from build123d import *

# Parameters (mm, degrees)
F1_DEPTH = 16


with BuildPart() as f1:
    # F0 (on Front) → F1 (new body)
    with BuildSketch(Plane.XZ):
        with BuildLine():
            ThreePointArc((0, 55), (16.109127, 16.109127), (55, 0))
            Line((55, 0), (195, 0))
            ThreePointArc((195, 0), (233.890873, 16.109127), (250, 55))
            Line((250, 55), (250, 545))
            ThreePointArc((250, 545), (233.890873, 583.890873), (195, 600))
            Line((195, 600), (125, 600))
            Line((125, 600), (90, 525))
            Line((90, 525), (0, 525))
            Line((0, 525), (0, 55))
        make_face()
        with BuildLine():
            ThreePointArc((48, 172), (50.928932, 179.071068), (58, 182))
            Line((58, 182), (190, 182))
            ThreePointArc((190, 182), (197.071068, 179.071068), (200, 172))
            Line((200, 172), (200, 40))
            ThreePointArc((200, 40), (197.071068, 32.928932), (190, 30))
            Line((190, 30), (58, 30))
            ThreePointArc((58, 30), (50.928932, 32.928932), (48, 40))
            Line((48, 40), (48, 172))
        make_face(mode=Mode.SUBTRACT)
    extrude(amount=F1_DEPTH)


solid = f1.part
Here's how the part is built. I have some questions about the finished solid (model axes, mm). A direction names the side the tool comes from. Give positions to 0.01 mm unless a question says otherwise; leave off trailing zeros. Order: outer loops, then holes, each group sorted by start corner. A loop starts at its lowest first (then second) coordinate and runs counter-clockwise, first axis right, second up. Notation, with made-up numbers: (-8, 77.25) -> (-2, 77.25) arc R15 ccw to (-2, 81.25) -> close; hole circle Ø11 at (-21.75, 2.5). An arc over 180 degrees is marked (long way). Use a Markdown table: item, result. Add a question column.
Item 1: Imagine slicing it at D-D on z = 533.5. Please give me the cut outline in (x, y).
Item 2: I need wall thicknesses on line 1 (Z direction, x = 63.5, y = -12.5); line 2 (Z direction, x = 174, y = -14.25); line 3 (X direction, y = -9.75, z = 35.5). Which ranges of each line are inside material? Lowest first, please.
Item 3: For faces 4 (the face through (123, 0, 304)), 5 (the face through (46, -8, 525)), 6 (the face through (125, -8, 30)), which set-ups out of +Z, -Z, +X, -X, +Y, -Y let a thin tool reach every point of the face, with its end or its side?
Item 4: If we mould it in two halves opening along X, with no side actions, what happens to faces 1 (the face through (160, -8, 600)), 2 (the face through (233.461, -7.888, 15.684)), 3 (the face through (197.15, -7.89, 33.01))? For each: pulls with the +X half, pulls with the -X half, needs draft (parallel to the pull), parting line crosses it, or undercut.
Item 5: Imagine slicing it at A-A on x = 77.5. Please give me the cut outline in (y, z), plus the area to 3 significant figures.
Item 6: Imagine slicing it at B-B on z = 99. Please give me the cut outline in (x, y).
Item 7: Imagine slicing it at C-C on y = -3.25. Please give me the cut outline in (x, z).
Item 8: Will these pins go through, and if not, where does the flat tip stop? pin 1 (1 mm diameter, centred on x = 119.5, y = -9, fed in from +Z); pin 2 (5 mm diameter, centred on x = 26, y = -7.5, fed in from +Z).
Data:
| question | item | result |
|---|---|---|
| 1 | outline | (93.97, -16) -> (250, -16) -> (250, 0) -> (93.97, 0) -> close |
| 2 | line 1 | z = 0 to 30, 182 to 525 |
| 2 | line 2 | z = 0 to 30, 182 to 600 |
| 2 | line 3 | x = 3.57 to 49.07, 198.93 to 246.43 |
| 3 | face 4 | +Z, -Z, +X, -X, +Y |
| 3 | face 5 | +Z, -X, +Y, -Y |
| 3 | face 6 | +Y, -Y |
| 4 | face 1 | needs draft |
| 4 | face 2 | pulls with the +X half |
| 4 | face 3 | undercut |
| 5 | outline | (-16, 0) -> (0, 0) -> (0, 30) -> (-16, 30) -> close; (-16, 182) -> (0, 182) -> (0, 525) -> (-16, 525) -> close |
| 5 | area | 5,970 mm² |
| 6 | outline | (0, -16) -> (48, -16) -> (48, 0) -> (0, 0) -> close; (200, -16) -> (250, -16) -> (250, 0) -> (200, 0) -> close |
| 7 | outline | (0, 55) arc R55 ccw to (55, 0) -> (195, 0) arc R55 ccw to (250, 55) -> (250, 545) arc R55 ccw to (195, 600) -> (125, 600) -> (90, 525) -> (0, 525) -> close; hole (48, 40) arc R10 ccw to (58, 30) -> (190, 30) arc R10 ccw to (200, 40) -> (200, 172) arc R10 ccw to (190, 182) -> (58, 182) arc R10 ccw to (48, 172) -> close |
| 8 | pin 1 | stops at z = 589.29 |
| 8 | pin 2 | stops at z = 525 |
